```python
from build123d import *

# Parameters (mm, degrees)
SKETCH012_R           = 93
PAD008_DEPTH          = 1.6
POCKET003_DEPTH       = 527.6981773351
POLARPATTERN001_COUNT = 4
SKETCH015_R           = 8
POCKET004_DEPTH       = 1.601
SKETCH013_R           = 8
PAD009_DEPTH          = 12
CHAMFER005_SIZE2      = 0.2
CHAMFER005_SIZE       = 3
CHAMFER006_SIZE       = 0.8


with BuildPart() as part:
    # Sketch012 → Pad008 (new body)
    with BuildSketch(Plane.XY):
        Circle(SKETCH012_R)
    extrude(amount=PAD008_DEPTH)

    # Sketch014 → Pocket003 (cut, through all)
    with BuildSketch(Plane.XY):
        with BuildLine():
            Line((-29.7321374946, 4), (-84.9058301885, 4))
            ThreePointArc((-62.8659154133, 57.2090611638), (-78.5297602635, 32.528091751), (-84.9058301885, 4))
            Line((-62.8659154133, 57.2090611638), (-23.8522231664, 18.1953689169))
            ThreePointArc((-23.8522231664, 18.1953689169), (-27.7163859753, 11.480502971), (-29.7321374946, 4))
        make_face()
        with BuildLine():
            Line((-18.1953689169, 23.8522231664), (-57.2090611638, 62.8659154133))
            ThreePointArc((-4, 84.9058301885), (-32.528091751, 78.5297602635), (-57.2090611638, 62.8659154133))
            Line((-4, 29.7321374946), (-4, 84.9058301885))
            ThreePointArc((-4, 29.7321374946), (-11.480502971, 27.7163859753), (-18.1953689169, 23.8522231664))
        make_face()
    pocket003 = extrude(amount=POCKET003_DEPTH, mode=Mode.SUBTRACT)

    # PolarPattern001: Pocket003 ×4 about axis
    polarpattern001_axis = Axis((0, 0, 0), (0, 0, 1))
    for i in range(1, POLARPATTERN001_COUNT):
        add(pocket003.rotate(polarpattern001_axis, i * 360 / POLARPATTERN001_COUNT), mode=Mode.SUBTRACT)

    # Sketch015 → Pocket004 (cut, through all)
    with BuildSketch(Plane.XY.offset(1.6)):
        Circle(SKETCH015_R)
    extrude(amount=-POCKET004_DEPTH, mode=Mode.SUBTRACT)

    # Sketch013 → Pad009 (join)
    with BuildSketch(Plane.XY.offset(1.6)):
        with BuildLine():
            ThreePointArc((-23.4, 0), (0, -23.4), (23.4, 0))
            ThreePointArc((23.9970767333, 0), (23.6985383667, 0.2704222444), (23.4, 0))
            ThreePointArc((17.6776695297, -17.6776695297), (22.8235419267, -9.5488497004), (23.9970767333, 0))
            ThreePointArc((-25, 0), (-9.5670858091, -23.0969883128), (17.6776695297, -17.6776695297))
            ThreePointArc((21.5, 0), (-1.75, 23.25), (-25, 0))
            ThreePointArc((-9.6, -2.3e-09), (5.9500000012, -15.5499999986), (21.5, 0))
            ThreePointArc((-5.6336134454, -7.7731846465), (8.5511019487, 4.3633307762), (-9.6, 0))
            ThreePointArc((-5.6336134454, -7.7731846465), (10.0127018373, -13.3452970661), (19.9, 0))
            ThreePointArc((19.9, 0), (-1.75, 21.65), (-23.4, 0))
        make_face()
        Circle(SKETCH013_R, mode=Mode.SUBTRACT)
        with BuildLine():
            ThreePointArc((-11.5, 0), (-16.5, 5), (-21.5, 0))
            ThreePointArc((-21.5, 0), (-8.6937875889, -19.6638769667), (14.4691216149, -15.90265763))
            ThreePointArc((14.4691216149, -15.90265763), (14.5126122143, -15.5081737413), (14.1266540458, -15.4157331507))
            ThreePointArc((-11.5, 0), (-3.0449954664, -14.9530116204), (14.1266540458, -15.4157331507))
        make_face()
    extrude(amount=PAD009_DEPTH)

    # Chamfer005
    chamfer005_edges = [part.edges().sort_by_distance(p)[0] for p in [
        (-8.693788, -19.663877, 13.6),
    ]]
    chamfer005_side = part.faces().sort_by_distance((-8.693788, -19.663877, 7.6))[0]
    chamfer(chamfer005_edges, length=CHAMFER005_SIZE, length2=CHAMFER005_SIZE2, reference=chamfer005_side)

    # Chamfer006
    chamfer006_edges = [part.edges().sort_by_distance(p)[0] for p in [
        (-8, 0, 13.6),
    ]]
    chamfer(chamfer006_edges, length=CHAMFER006_SIZE)


solid = part.part
```
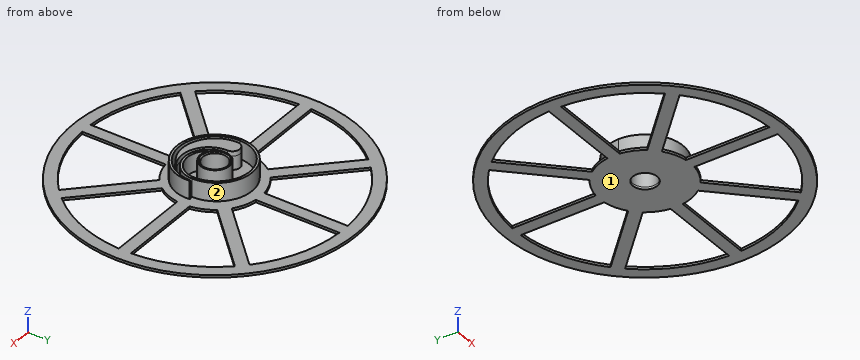
CAD build for the part. Positions are in the model's coordinates, mm. Face numbers are marked on the shaded views. A direction names the side the tool comes from. Coordinates: 2 decimals unless noted, no trailing zeros. Order: outer loops, then holes, each group sorted by start corner. A loop starts at its lowest first (then second) coordinate and runs counter-clockwise, first axis right, second up. Notation, with made-up numbers: (20.5, -11.5) - (63.5, -11.5) arc R33 cw to (63.5, 17.5) - close; hole circle Ø11 at (-32.5, 12.25). An arc over 180 degrees is marked (long way). Use a Markdown table: item, result. Add a question column.
(1) Flat gauge pins, fed straight in: pin 1 (1.3 mm diameter, centred on y = 62, z = 0.5, fed in from +X); pin 2 (1.3 mm diameter, centred on x = 55, z = 0.5, fed in from -Y); pin 3 (0.5 mm diameter, centred on x = -49, z = 0.5, fed in from -Y). Where does each tip first touch, or does it go through?
(2) Which spindle directions (+Z, -Z, +X, -X, +Y, -Y) get a long thin tool onto all of the face, cutting with end or side? Do the marked faces 1 and 2. Say none if no direction does.
(3) Drill centre lines: line 1 along Y through (x, z) = (0, 4.5); line 2 along X through (y, z) = (-6, 1.25); line 3 along Y through (x, z) = (-18, 1). Where is each one in solid material? Low to high. Write a range as [from, to].
(4) Saw through at B-B (x = -68). Give the cut face in (y, z), then the cut area to 3 significant figures.
(5) Saw through at A-A (z = 4.5). Give the cut face in (x, y), then the cut area to 3 significant figures.
Solved:
| question | item | result |
|---|---|---|
| 1 | pin 1 | stops at x = 69.89 |
| 1 | pin 2 | stops at y = -75.47 |
| 1 | pin 3 | stops at y = -79.2 |
| 2 | face 1 | -Z, +X, -X, +Y, -Y |
| 2 | face 2 | +Z, +Y |
| 3 | line 1 | y = [-25, -23.4], [-21.5, -16.4], [-14.37, -12.62], [-9.6, -8], [8, 9.6], [21.58, 23.18] |
| 3 | line 2 | x = [-92.81, -84.79], [-29.39, -5.29], [5.29, 29.39], [84.79, 92.81] |
| 3 | line 3 | y = [-91.24, -83.07], [-24, 24], [83.07, 91.24] |
| 4 | outline | (-63.44, 0) - (-51, 0) - (-51, 1.6) - (-63.44, 1.6) - close; (-4, 0) - (4, 0) - (4, 1.6) - (-4, 1.6) - close; (51, 0) - (63.44, 0) - (63.44, 1.6) - (51, 1.6) - close |
| 4 | area | 52.6 mm² |
| 5 | outline | (-25, 0) arc R25 ccw to (17.68, -17.68) arc R21.94 ccw to (24, 0) arc R0.3 ccw to (23.4, 0) arc R23.4 cw to (-23.4, 0) arc R21.65 cw to (19.9, 0) arc R13.95 cw to (-5.63, -7.77) arc R9.6 ccw (long way) to (-9.6, 0) arc R15.55 ccw to (21.5, 0) arc R23.25 ccw to start; (-21.5, 0) arc R21.5 ccw to (14.47, -15.9) arc R0.3 ccw to (14.13, -15.42) arc R17.45 cw to (-11.5, 0) arc R5 ccw to start; hole circle Ø16 at (0, 0) |
| 5 | area | 688 mm² |
